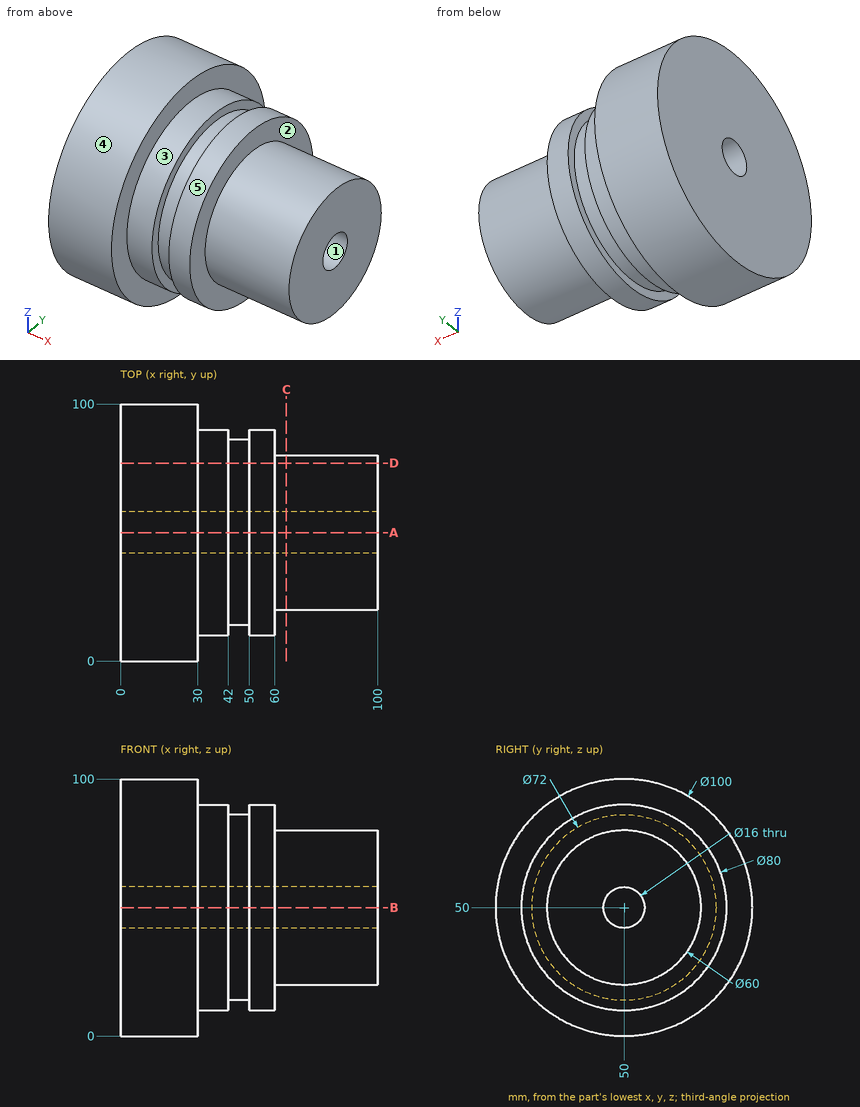
Job drawing, mm, ordinate dimensions from the low corner. One solid piece. A direction names the side the tool comes from. Round coordinates to 2 decimals unless told otherwise and drop trailing zeros. Write each loop counter-clockwise with the first axis right and the second up, starting at its lowest first coordinate (ties: lowest second). Pieces come first, ordered by that corner, then holes. Notation, with made-up numbers: M -26.5,17 L -11.5,17 A19 ccw -11.5,32 Z; hole C 79,-11.5 d8. An arc over 180 degrees is marked long. Return JSON: item names as keys, results as strings. Group by question number.
(1) Which spindle directions (+Z, -Z, +X, -X, +Y, -Y) get a long thin tool onto all of the face, cutting with end or side? Do the marked faces 4 and 5. Say none if no direction does.
(2) Saw through at D-D on y = 77. Write the cut outline in (x, z).
(3) Saw through at C-C on x = 64.5. Write the cut outline in (y, z).
(4) Pin check, flat tips, straight feed: pin 1 Ø8 at (x, y) = (54.5, 22) entering from -Z; pin 2 Ø4 at (x, y) = (26.5, 19) entering from +Z; pin 3 Ø10 at (x, z) = (88.5, 51) entering from +Y. Stop position of each tip, or through.
(5) Two-plate mould, pull along Z, no slides. Class the marked faces 1, 2 and 3: +Z half, -Z half, draft (parallel to the pull), parting line (faces both ways), or undercut.
(6) Saw through at A-A on y = 50. Write the cut outline in (x, z), then the cut area to 3 significant figures.
(7) Drill centre lines: probe 1 along Z at (x, y) = (48.5, 50.5); probe 2 along Z at (x, y) = (41, 50); probe 3 along X at (y, z) = (91, 78). Where is each one in solid material? Low to high.
Returned:
{
 "1": {"face 4": "+X, -X", "face 5": "+X"},
 "2": {"outline": "M 0,7.92 L 30,7.92 L 30,20.49 L 42,20.49 L 42,26.19 L 50,26.19 L 50,20.49 L 60,20.49 L 60,36.92 L 100,36.92 L 100,63.08 L 60,63.08 L 60,79.51 L 50,79.51 L 50,73.81 L 42,73.81 L 42,79.51 L 30,79.51 L 30,92.08 L 0,92.08 Z"},
 "3": {"outline": "C 50,50 d60; hole C 50,50 d16"},
 "4": {"pin 1": "z = 18", "pin 2": "z = 90.73", "pin 3": "y = 80"},
 "5": {"face 1": "undercut", "face 2": "draft", "face 3": "parting line"},
 "6": {"outline": "M 0,0 L 30,0 L 30,10 L 42,10 L 42,14 L 50,14 L 50,10 L 60,10 L 60,20 L 100,20 L 100,42 L 0,42 Z; M 0,58 L 100,58 L 100,80 L 60,80 L 60,90 L 50,90 L 50,86 L 42,86 L 42,90 L 30,90 L 30,100 L 0,100 Z", "area": "6,140 mm²"},
 "7": {"probe 1": "14 to 42.02, 57.98 to 86", "probe 2": "10 to 42, 58 to 90", "probe 3": "0 to 30"}
}
